Could you check a few things on this model? Use its own coordinates, in mm. Face numbers are marked on the shaded views. A direction names the side the tool comes from. Coordinates: 2 decimals unless noted, no trailing zeros. Order: outer loops, then holes, each group sorted by start corner. A loop starts at its lowest first (then second) coordinate and runs counter-clockwise, first axis right, second up. Notation, with made-up numbers: (-24, 22) - (23, 22) arc R22 cw to (23, 43) - close; hole circle Ø2 at (-36, 72.25). An arc over 180 degrees is marked (long way). Answer as CSV lines item,"result". Start each with the question number.
1. I want a section at B-B, the plane z = -47.5. List the corners of the cut face in (x, y) for me.
2. Thinking about a two-plate mould opening in X: for the marked faces 3, 4 and 5, which applies, released by +X, released by -X, zero draft, split by the parting line, or undercut?
3. I need wall thicknesses on probe 1 along X at (y, z) = (33.5, -131); probe 2 along Y at (x, z) = (168, -20). Which ranges of each line are inside material? Lowest first, please.
4. For the marked faces 1 and 2, which set-ups out of +Z, -Z, +X, -X, +Y, -Y let a thin tool reach every point of the face, with its end or its side?
5. I want a section at A-A, the plane y = 16. List the corners of the cut face in (x, z) for me, and give its area (3 significant figures).
6. For pin 1 (2 mm diameter, centred on x = 215.5, y = 8.5, fed in from -Z); pin 2 (3 mm diameter, centred on x = 147.5, z = -177, fed in from +Y), each with a flat end and sliding along its axis, tell me the tip position at first contact or that it passes through.
7. I want a section at C-C, the plane x = 122. List the corners of the cut face in (y, z) for me, and give its area (3 significant figures).
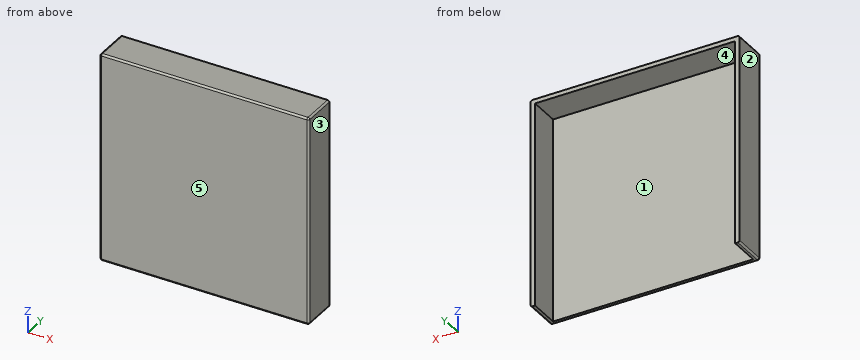
from build123d import *

# Parameters (mm, degrees)
SKETCH1_W           = 304.8
SKETCH1_H           = 304.8
BOSS_EXTRUDE1_DEPTH = 50.8
SHELL1_T            = -6.35
FILLET1_R           = 2.54


with BuildPart() as part:
    # Sketch1 → Boss-Extrude1 (new body)
    with BuildSketch(Plane(origin=(0, 0, 0), x_dir=(1, 0, 0), z_dir=(0, 1, 0))):
        with Locations((152.4, 152.4)):
            Rectangle(SKETCH1_W, SKETCH1_H)
    extrude(amount=BOSS_EXTRUDE1_DEPTH)

    # Shell1
    shell1_openings = [part.faces().sort_by_distance(p)[0] for p in [
        (152.4, 50.8, -152.4),
        (152.4, 25.4, -304.8),
    ]]
    offset(amount=SHELL1_T, openings=shell1_openings, kind=Kind.INTERSECTION)

    # Fillet1
    fillet1_edges = [part.edges().sort_by_distance(p)[0] for p in [
        (152.4, 0, -304.8),
        (304.8, 0, -152.4),
        (152.4, 0, 0),
        (0, 0, -152.4),
        (0, 25.4, -304.8),
        (304.8, 25.4, -304.8),
        (304.8, 25.4, 0),
        (0, 25.4, 0),
    ]]
    fillet(fillet1_edges, radius=FILLET1_R)


solid = part.part
Solved:
1,outline,"(0, 2.54) arc R2.54 ccw to (2.54, 0) - (302.26, 0) arc R2.54 ccw to (304.8, 2.54) - (304.8, 50.8) - (298.45, 50.8) - (298.45, 6.35) - (6.35, 6.35) - (6.35, 50.8) - (0, 50.8) - close"
2,face 3,"released by +X"
2,face 4,"undercut"
2,face 5,"zero draft"
3,probe 1,"x = 0 to 6.35, 298.45 to 304.8"
3,probe 2,"y = 0 to 6.35"
4,face 1,"-Z, +Y"
4,face 2,"+Z, -Z, -X, +Y, -Y"
5,outline,"(0, -302.26) arc R2.54 ccw to (2.54, -304.8) - (6.35, -304.8) - (6.35, -6.35) - (298.45, -6.35) - (298.45, -304.8) - (302.26, -304.8) arc R2.54 ccw to (304.8, -302.26) - (304.8, -2.54) arc R2.54 ccw to (302.26, 0) - (2.54, 0) arc R2.54 ccw to (0, -2.54) - close"
5,area,"5,720 mm2"
6,pin 1,"stops at z = -6.35"
6,pin 2,"stops at y = 6.35"
7,outline,"(0, -302.26) arc R2.54 ccw to (2.54, -304.8) - (6.35, -304.8) - (6.35, -6.35) - (50.8, -6.35) - (50.8, 0) - (2.54, 0) arc R2.54 ccw to (0, -2.54) - close"
7,area,"2,210 mm2"
